Work out the finished part from the listing and answer in its coordinate system (mm). Face numbers are marked on the shaded views. A direction names the side the tool comes from. Give positions to 0.01 mm unless a question says otherwise; leave off trailing zeros. Write each loop counter-clockwise with the first axis right and the second up, starting at its lowest first coordinate (ties: lowest second). Pieces come first, ordered by that corner, then holes.
1) Find section B-B (x = -23). Determine the outline of the cut face in (y, z).
2) Find section A-A (z = -1.5). Determine the outline of the cut face in (x, y).
3) Find section D-D (z = 7). Determine the outline of the cut face in (x, y).
4) Determine the mould class of the marked faces 1, 2 and 3 for opening direction Z: pulls with the +Z half, pulls with the -Z half, needs draft (parallel to the pull), parting line crosses it, or undercut.
5) Given pin 1 Ø5 at (y, z) = (-12.99, -7.5) entering from +X; pin 2 Ø0.9 at (y, z) = (-13.5, -8) entering from +X; pin 3 Ø1.5 at (x, z) = (-24.5, -8) entering from -Y, each flat-ended and moving along its own axis, determine where each tip first touches the part or whether it passes through.
6) Find section C-C (y = -6). Determine the outline of the cut face in (x, z), plus the area to 3 significant figures.
7) Straight lines are drawn through the part: probe 1 along Y at (x, z) = (18, 7); probe 2 along Y at (x, z) = (19.05, 7.5); probe 3 along Y at (x, z) = (21, 0). For each, find the intervals that lie inside material, in ascending order.
8) A tool of negligible diameter and unlimited length cuts with its end or side. For the marked faces 4, 5 and 6, from which of +Z, -Z, +X, -X, +Y, -Y can it reach the whole face along a straight path? Write none if from no direction.
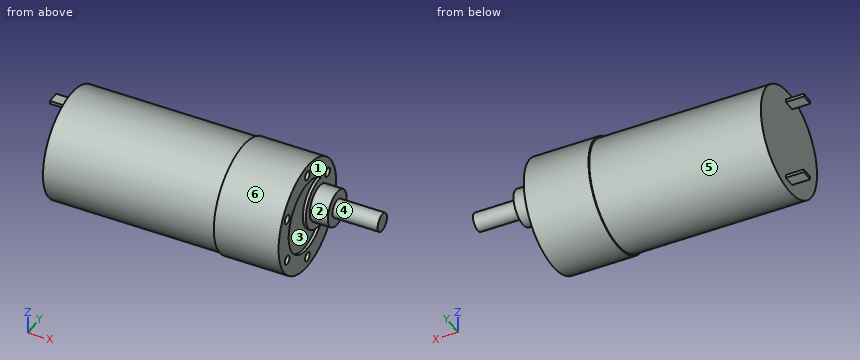
```python
from build123d import *

# Parameters (mm, degrees)
SKETCH1_R           = 18.5
BOSS_EXTRUDE1_DEPTH = 21.5
SKETCH2_R           = 18
BOSS_EXTRUDE2_DEPTH = 57
SKETCH3_W           = 1
SKETCH3_H           = 4
BOSS_EXTRUDE3_DEPTH = 6
SKETCH4_R           = 6
BOSS_EXTRUDE4_DEPTH = 6
SKETCH5_R           = 3
BOSS_EXTRUDE5_DEPTH = 15
CUT_EXTRUDE1_DEPTH  = 1
SKETCH7_R           = 1.5
CUT_EXTRUDE2_DEPTH  = 5


with BuildPart() as part:
    # Sketch1 → Boss-Extrude1 (new body)
    with BuildSketch(Plane(origin=(0, 0, 0), x_dir=(0, 0, -1), z_dir=(1, 0, 0))):
        Circle(SKETCH1_R)
    extrude(amount=BOSS_EXTRUDE1_DEPTH)

    # Sketch2 → Boss-Extrude2 (add)
    with BuildSketch(Plane.ZY):
        Circle(SKETCH2_R)
    extrude(amount=BOSS_EXTRUDE2_DEPTH)

    # Sketch3 → Boss-Extrude3 (add)
    with BuildSketch(Plane.ZY.offset(57)):
        with Locations((-14, 0)):
            Rectangle(SKETCH3_W, SKETCH3_H)
        with Locations((14, 0)):
            Rectangle(SKETCH3_W, SKETCH3_H)
    extrude(amount=BOSS_EXTRUDE3_DEPTH)

    # Sketch4 → Boss-Extrude4 (add)
    with BuildSketch(Plane(origin=(21.5, 0, 0), x_dir=(0, 0, -1), z_dir=(1, 0, 0))):
        with Locations((0, 7.5)):
            Circle(SKETCH4_R)
    extrude(amount=BOSS_EXTRUDE4_DEPTH)

    # Sketch5 → Boss-Extrude5 (add)
    with BuildSketch(Plane(origin=(27.5, 0, 0), x_dir=(0, 0, -1), z_dir=(1, 0, 0))):
        with Locations((0, 7.5)):
            Circle(SKETCH5_R)
    extrude(amount=BOSS_EXTRUDE5_DEPTH)

    # Sketch6 → Cut-Extrude1 (cut)
    with BuildSketch(Plane(origin=(21.5, 0, 0), x_dir=(0, 0, -1), z_dir=(1, 0, 0))):
        with BuildLine():
            ThreePointArc((-8.436955744, 8.533333333), (-4.623663649, -11.073469847), (12, 0))
            ThreePointArc((12, 0), (11.073469847, 4.623663649), (8.436955744, 8.533333333))
            ThreePointArc((8.436955744, 8.533333333), (8.484224296, 8.017627365), (8.5, 7.5))
            ThreePointArc((8.5, 7.5), (-0.517627365, -0.984224296), (-8.436955744, 8.533333333))
        make_face()
    extrude(amount=-CUT_EXTRUDE1_DEPTH, mode=Mode.SUBTRACT)

    # Sketch7 → Cut-Extrude2 (cut)
    with BuildSketch(Plane(origin=(21.5, 0, 0), x_dir=(0, 0, -1), z_dir=(1, 0, 0))):
        with Locations((-15, 0)):
            Circle(SKETCH7_R)
        with Locations((-7.5, 12.990381057)):
            Circle(SKETCH7_R)
        with Locations((7.5, 12.990381057)):
            Circle(SKETCH7_R)
        with Locations((15, 0)):
            Circle(SKETCH7_R)
        with Locations((7.5, -12.990381057)):
            Circle(SKETCH7_R)
        with Locations((-7.5, -12.990381057)):
            Circle(SKETCH7_R)
    extrude(amount=-CUT_EXTRUDE2_DEPTH, mode=Mode.SUBTRACT)


solid = part.part
```
Results:
1. outline: circle Ø36 at (0, 0)
2. outline: (-57, -17.94) - (0, -17.94) - (0, -18.44) - (21.5, -18.44) - (21.5, -11.91) - (20.5, -11.91) - (20.5, -0.87) - (21.5, -0.87) - (21.5, 1.69) - (27.5, 1.69) - (27.5, 4.9) - (42.5, 4.9) - (42.5, 10.1) - (27.5, 10.1) - (27.5, 13.31) - (21.5, 13.31) - (21.5, 18.44) - (0, 18.44) - (0, 17.94) - (-57, 17.94) - close
3. outline: (-57, -16.58) - (0, -16.58) - (0, -17.12) - (21.5, -17.12) - (21.5, -14.4) - (16.5, -14.4) - (16.5, -11.58) - (21.5, -11.58) - (21.5, -9.75) - (20.5, -9.75) - (20.5, 2.68) - (21.5, 2.68) - (21.5, 11.58) - (16.5, 11.58) - (16.5, 14.4) - (21.5, 14.4) - (21.5, 17.12) - (0, 17.12) - (0, 16.58) - (-57, 16.58) - close
4. face 1: needs draft
4. face 2: parting line crosses it
4. face 3: undercut
5. pin 1: stops at x = 21.5
5. pin 2: stops at x = 16.5
5. pin 3: stops at y = -16.48
6. outline: (-57, -16.97) - (0, -16.97) - (0, -17.5) - (21.5, -17.5) - (21.5, -10.39) - (20.5, -10.39) - (20.5, 10.39) - (21.5, 10.39) - (21.5, 17.5) - (0, 17.5) - (0, 16.97) - (-57, 16.97) - close
6. area: 2,670 mm2
7. probe 1: y = -17.12 to -14.4, -11.58 to 11.58, 14.4 to 17.12
7. probe 2: y = -16.91 to -14.49, -11.49 to 11.49, 14.49 to 16.91
7. probe 3: y = -18.5 to -12, -1 to 18.5
8. face 4: +X
8. face 5: -X
8. face 6: +X, -X
